```python
from build123d import *

# Parameters (mm, degrees)
SKETCH1_R           = 110
SKETCH1_R_2         = 4.25
SKETCH1_R_3         = 15.5
BOSS_EXTRUDE1_DEPTH = 6
CUT_EXTRUDE1_START  = -2
CUT_EXTRUDE1_DEPTH  = 6
BOSS_EXTRUDE3_START = -6
SKETCH4_W           = 10
SKETCH4_H           = 10
BOSS_EXTRUDE3_DEPTH = 76


with BuildPart() as part:
    # Sketch1 → Boss-Extrude1 (new body)
    with BuildSketch(Plane(origin=(0, 0, 0), x_dir=(1, 0, 0), z_dir=(0, 1, 0))):
        with Locations(Location((0, 0, 0), (0, 0, 270))):
            Circle(SKETCH1_R)
        with Locations(Location((-90, 0, 0), (0, 0, 270))):
            Circle(SKETCH1_R_2, mode=Mode.SUBTRACT)
        with Locations(Location((-84.572335871, 30.781812899, 0), (0, 0, 270))):
            Circle(SKETCH1_R_2, mode=Mode.SUBTRACT)
        with Locations(Location((-68.943999881, 57.850884872, 0), (0, 0, 270))):
            Circle(SKETCH1_R_2, mode=Mode.SUBTRACT)
        with Locations(Location((-45, 77.942286341, 0), (0, 0, 270))):
            Circle(SKETCH1_R_2, mode=Mode.SUBTRACT)
        with Locations(Location((-15.62833599, 88.632697771, 0), (0, 0, 270))):
            Circle(SKETCH1_R_2, mode=Mode.SUBTRACT)
        with Locations(Location((15.62833599, 88.632697771, 0), (0, 0, 270))):
            Circle(SKETCH1_R_2, mode=Mode.SUBTRACT)
        with Locations(Location((45, 77.942286341, 0), (0, 0, 270))):
            Circle(SKETCH1_R_2, mode=Mode.SUBTRACT)
        with Locations(Location((68.943999881, 57.850884872, 0), (0, 0, 270))):
            Circle(SKETCH1_R_2, mode=Mode.SUBTRACT)
        with Locations(Location((84.572335871, 30.781812899, 0), (0, 0, 270))):
            Circle(SKETCH1_R_2, mode=Mode.SUBTRACT)
        with Locations(Location((90, 0, 0), (0, 0, 270))):
            Circle(SKETCH1_R_2, mode=Mode.SUBTRACT)
        with Locations(Location((84.572335871, -30.781812899, 0), (0, 0, 270))):
            Circle(SKETCH1_R_2, mode=Mode.SUBTRACT)
        with Locations(Location((68.943999881, -57.850884872, 0), (0, 0, 270))):
            Circle(SKETCH1_R_2, mode=Mode.SUBTRACT)
        with Locations(Location((45, -77.942286341, 0), (0, 0, 270))):
            Circle(SKETCH1_R_2, mode=Mode.SUBTRACT)
        with Locations(Location((15.62833599, -88.632697771, 0), (0, 0, 270))):
            Circle(SKETCH1_R_2, mode=Mode.SUBTRACT)
        with Locations(Location((-15.62833599, -88.632697771, 0), (0, 0, 270))):
            Circle(SKETCH1_R_2, mode=Mode.SUBTRACT)
        with Locations(Location((-45, -77.942286341, 0), (0, 0, 270))):
            Circle(SKETCH1_R_2, mode=Mode.SUBTRACT)
        with Locations(Location((-68.943999881, -57.850884872, 0), (0, 0, 270))):
            Circle(SKETCH1_R_2, mode=Mode.SUBTRACT)
        with Locations(Location((-84.572335871, -30.781812899, 0), (0, 0, 270))):
            Circle(SKETCH1_R_2, mode=Mode.SUBTRACT)
        with Locations(Location((0, 0, 0), (0, 0, 270))):
            Circle(SKETCH1_R_3, mode=Mode.SUBTRACT)
    extrude(amount=BOSS_EXTRUDE1_DEPTH)

    # Sketch2 → Cut-Extrude1 (cut)
    with BuildSketch(Plane(origin=(0, 6, 0), x_dir=(1, 0, 0), z_dir=(0, 1, 0)).offset(CUT_EXTRUDE1_START)):
        Polygon((-87.034881158, 24.016026123), (-79.944265289, 25.266292734), (-77.481720002, 32.032079511), (-82.109790583, 37.547599676), (-89.200406452, 36.297333065), (-91.66295174, 29.531546288), align=None)
        Polygon((-90.000000272, -7.2), (-83.764617229, -3.600000236), (-83.764616957, 3.599999764), (-89.999999728, 7.2), (-96.235382771, 3.600000236), (-96.235383043, -3.599999764), align=None)
        Polygon((-73.572070879, 52.335365056), (-66.481455104, 51.085097909), (-61.853384106, 56.600617725), (-64.315928883, 63.366404687), (-71.406544657, 64.616671834), (-76.034615655, 59.101152019), align=None)
        Polygon((-51.235383043, 74.342286576), (-45.000000272, 70.742286341), (-38.764617229, 74.342286105), (-38.764616957, 81.542286105), (-44.999999728, 85.142286341), (-51.235382771, 81.542286576), align=None)
        Polygon((-22.718951859, 87.38243116), (-18.090881278, 81.866910994), (-11.000265409, 83.117177606), (-8.537720121, 89.882964382), (-13.165790702, 95.398484548), (-20.256406571, 94.148217936), align=None)
        Polygon((8.537720216, 89.882964918), (11.000264992, 83.117177955), (18.090880766, 81.866910808), (22.718951764, 87.382430624), (20.256406988, 94.148217587), (13.165791214, 95.398484734), align=None)
        Polygon((38.764617229, 81.542286576), (38.764616957, 74.342286576), (44.999999728, 70.742286341), (51.235382771, 74.342286105), (51.235383043, 81.542286105), (45.000000272, 85.142286341), align=None)
        Polygon((64.315929299, 63.366405037), (61.853384012, 56.60061826), (66.481454593, 51.085098095), (73.572070462, 52.335364706), (76.03461575, 59.101151483), (71.406545168, 64.616671648), align=None)
        Polygon((82.109791094, 37.547599862), (77.481720096, 32.032080046), (79.944264873, 25.266293084), (87.034880647, 24.016025937), (91.662951645, 29.531545752), (89.200406869, 36.297332715), align=None)
        Polygon((90.000000272, 7.2), (83.764617229, 3.600000236), (83.764616957, -3.599999764), (89.999999728, -7.2), (96.235382771, -3.600000236), (96.235383043, 3.599999764), align=None)
        Polygon((87.034881158, -24.016026123), (79.944265289, -25.266292734), (77.481720002, -32.032079511), (82.109790583, -37.547599676), (89.200406452, -36.297333065), (91.66295174, -29.531546288), align=None)
        Polygon((73.572070879, -52.335365056), (66.481455104, -51.085097909), (61.853384106, -56.600617725), (64.315928883, -63.366404687), (71.406544657, -64.616671834), (76.034615655, -59.101152019), align=None)
        Polygon((51.235383043, -74.342286576), (45.000000272, -70.742286341), (38.764617229, -74.342286105), (38.764616957, -81.542286105), (44.999999728, -85.142286341), (51.235382771, -81.542286576), align=None)
        Polygon((22.718951859, -87.38243116), (18.090881278, -81.866910994), (11.000265409, -83.117177606), (8.537720121, -89.882964382), (13.165790702, -95.398484548), (20.256406571, -94.148217936), align=None)
        Polygon((-8.537720216, -89.882964918), (-11.000264992, -83.117177955), (-18.090880766, -81.866910808), (-22.718951764, -87.382430624), (-20.256406988, -94.148217587), (-13.165791214, -95.398484734), align=None)
        Polygon((-38.764617229, -81.542286576), (-38.764616957, -74.342286576), (-44.999999728, -70.742286341), (-51.235382771, -74.342286105), (-51.235383043, -81.542286105), (-45.000000272, -85.142286341), align=None)
        Polygon((-64.315929299, -63.366405037), (-61.853384012, -56.60061826), (-66.481454593, -51.085098095), (-73.572070462, -52.335364706), (-76.03461575, -59.101151483), (-71.406545168, -64.616671648), align=None)
        Polygon((-82.109791094, -37.547599862), (-77.481720096, -32.032080046), (-79.944264873, -25.266293084), (-87.034880647, -24.016025937), (-91.662951645, -29.531545752), (-89.200406869, -36.297332715), align=None)
    extrude(amount=-CUT_EXTRUDE1_DEPTH, mode=Mode.SUBTRACT)

    # Sketch4 → Boss-Extrude3 (add)
    with BuildSketch(Plane(origin=(0, 6, 0), x_dir=(1, 0, 0), z_dir=(0, 1, 0)).offset(BOSS_EXTRUDE3_START)):
        with Locations((-114.438621766, 0)):
            Rectangle(SKETCH4_W, SKETCH4_H)
        with Locations((114.438621766, 0)):
            Rectangle(SKETCH4_W, SKETCH4_H)
        with Locations((0, -114.438621766)):
            Rectangle(SKETCH4_W, SKETCH4_H)
        with Locations((0, 114.438621766)):
            Rectangle(SKETCH4_W, SKETCH4_H)
    extrude(amount=BOSS_EXTRUDE3_DEPTH)


solid = part.part
```
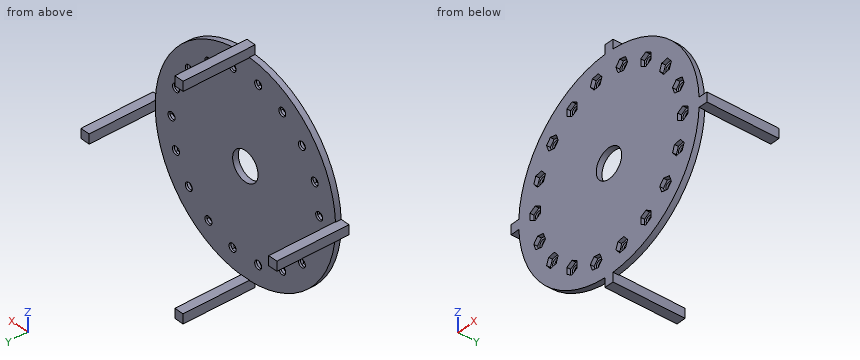
Can you work these out from the model? Positions are in its coordinate system, mm. Coordinates: 2 decimals unless noted, no trailing zeros. Loops run counter-clockwise (first coordinate to the right, second up) from the corner with the lowest first, then second, coordinate; pieces in that order, holes last. Notation, with made-up numbers: (11.25, 75.25) -> (25.25, 75.25) arc R24 cw to (25.25, 97.25) -> close; hole circle Ø9 at (-25.75, 14.5). An arc over 180 degrees is marked (long way). Answer as a JSON object with one key per item and string values.
1) Imagine slicing it at C-C (z = 42.5). Please give me the cut outline in (x, y), then the cut area to 3 significant figures.
Results:
{"outline": "(-101.46, 0) -> (101.46, 0) -> (101.46, 6) -> (-101.46, 6) -> close", "area": "1,220 mm^2"}
2) Imagine slicing it at A-A (y = 63.5). Please give me the cut outline in (x, z), then the cut area to 3 significant figures.
Results:
{"outline": "(-119.44, -5) -> (-109.44, -5) -> (-109.44, 5) -> (-119.44, 5) -> close; (-5, -119.44) -> (5, -119.44) -> (5, -109.44) -> (-5, -109.44) -> close; (-5, 109.44) -> (5, 109.44) -> (5, 119.44) -> (-5, 119.44) -> close; (109.44, -5) -> (119.44, -5) -> (119.44, 5) -> (109.44, 5) -> close", "area": "400 mm^2"}
3) For P1, Ø3, axis at x = -113.5, y = 23, coming from the +Z side; P2, Ø7.5, axis at x = 68.94, z = -57.85, coming from the +Y side; P3, Ø6, axis at x = 89, z = -3.5, coming from the -Y side; P4, Ø7, axis at x = -68, z = 57, coming from the -Y side, each with a flat end and sliding along its axis, tell me the tip position at first contact or that it passes through.
Results:
{"P1": "stops at z = 5", "P2": "passes through", "P3": "stops at y = 0", "P4": "stops at y = 4"}
4) Imagine slicing it at B-B (x = 0). Please give me the cut outline in (y, z), then the cut area to 3 significant figures.
Results:
{"outline": "(0, -119.44) -> (76, -119.44) -> (76, -109.44) -> (6, -109.44) -> (6, -15.5) -> (0, -15.5) -> close; (0, 15.5) -> (6, 15.5) -> (6, 109.44) -> (76, 109.44) -> (76, 119.44) -> (0, 119.44) -> close", "area": "2,650 mm^2"}
5) If I drill on line 1 (Z direction, x = 4.5, y = 58.5); line 2 (Y direction, x = 5, z = -16); line 3 (Z direction, x = -45, y = 5.25), over which ranges is the centre line in solid material (lowest first)?
Results:
{"line 1": "z = -119.44 to -109.44, 109.44 to 119.44", "line 2": "y = 0 to 6", "line 3": "z = -100.37 to -82.19, -73.69 to 73.69, 82.19 to 100.37"}
6) Imagine slicing it at D-D (x = -103). Please give me the cut outline in (y, z).
Results:
{"outline": "(0, -38.61) -> (6, -38.61) -> (6, 38.61) -> (0, 38.61) -> close"}
